Could you check a few things on this model? Use its own coordinates, in mm. Face numbers are marked on the shaded views. A direction names the side the tool comes from. Give positions to 0.01 mm unless a question says otherwise; leave off trailing zeros. Order: outer loops, then holes, each group sorted by start corner. A loop starts at its lowest first (then second) coordinate and runs counter-clockwise, first axis right, second up. Notation, with made-up numbers: (9, 45) -> (54, 45) arc R20 ccw to (54, 58) -> close; hole circle Ø3 at (-8.75, 49.5). An arc over 180 degrees is marked (long way). Answer as CSV lines item,"result". Start each with the question number.
(1) Will this pin go through, and if not, where does the flat tip stop? pin 1 Ø5 at (x, y) = (24, -1.5) entering from -Z.
(2) On a 3-axis mill with a long thin cutter (end or side, diameter ignored), from which of +Z, -Z, +X, -X, +Y, -Y can I reach the whole of each face in a straight line? I mean the marked faces 4 and 5. Say none if no direction works.
(3) I want a section at A-A (x = -8.5). Please give me the cut outline in (y, z).
(4) I want a section at C-C (z = 8.5). Please give me the cut outline in (x, y), plus the area to 4 significant figures.
(5) I want a section at B-B (y = -2). Please give me the cut outline in (x, z).
(6) We'd pull the mould along X, two halves only. Please class the marked faces 1, 2 and 3: released by +X, released by -X, zero draft, split by the parting line, or undercut.
(7) I need wall thicknesses on L1, parallel to X at y = 1, z = 2.75; L2, parallel to X at y = 6, z = 6; L3, parallel to Y at x = -19.5, z = 2. Which ranges of each line are inside material? Lowest first, please.
```python
from build123d import *

# Parameters (mm, degrees)
F0_W     = 67
F0_H     = 20
F0_W_2   = 5
F0_H_2   = 9
F0_H_3   = 10.5
F1_DEPTH = 10


with BuildPart() as f1:
    # F0 (on Top) → F1 (new body)
    with BuildSketch(Plane.XY):
        with Locations((2.5, 1.031276)):
            Rectangle(F0_W, F0_H)
        with Locations((26.5, 0.531276)):
            Rectangle(F0_W_2, F0_H_2, mode=Mode.SUBTRACT)
        with Locations((-21.5, 1.281276)):
            Rectangle(F0_W_2, F0_H_3, mode=Mode.SUBTRACT)
        with Locations((-9.5, 1.281276)):
            Rectangle(F0_W_2, F0_H_3, mode=Mode.SUBTRACT)
        with Locations((2.5, 1.281276)):
            Rectangle(F0_W_2, F0_H_3, mode=Mode.SUBTRACT)
        with Locations((14.5, 1.281276)):
            Rectangle(F0_W_2, F0_H_3, mode=Mode.SUBTRACT)
    extrude(amount=F1_DEPTH)


solid = f1.part
```
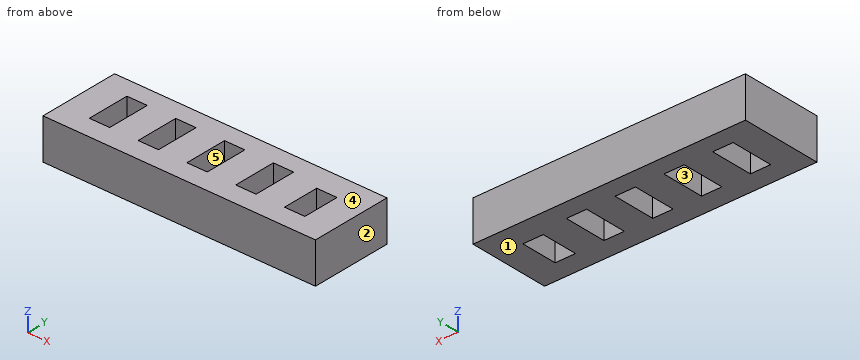
Final values:
1,pin 1,"z = 0"
2,face 4,"+Z, +X, -X, +Y, -Y"
2,face 5,"+Z, -Z"
3,outline,"(-8.97, 0) -> (-3.97, 0) -> (-3.97, 10) -> (-8.97, 10) -> close; (6.53, 0) -> (11.03, 0) -> (11.03, 10) -> (6.53, 10) -> close"
4,outline,"(-31, -8.97) -> (36, -8.97) -> (36, 11.03) -> (-31, 11.03) -> close; hole (-24, -3.97) -> (-19, -3.97) -> (-19, 6.53) -> (-24, 6.53) -> close; hole (-12, -3.97) -> (-7, -3.97) -> (-7, 6.53) -> (-12, 6.53) -> close; hole (0, -3.97) -> (5, -3.97) -> (5, 6.53) -> (0, 6.53) -> close; hole (12, -3.97) -> (17, -3.97) -> (17, 6.53) -> (12, 6.53) -> close; hole (24, -3.97) -> (29, -3.97) -> (29, 5.03) -> (24, 5.03) -> close"
4,area,"1,085 mm²"
5,outline,"(-31, 0) -> (-24, 0) -> (-24, 10) -> (-31, 10) -> close; (-19, 0) -> (-12, 0) -> (-12, 10) -> (-19, 10) -> close; (-7, 0) -> (0, 0) -> (0, 10) -> (-7, 10) -> close; (5, 0) -> (12, 0) -> (12, 10) -> (5, 10) -> close; (17, 0) -> (24, 0) -> (24, 10) -> (17, 10) -> close; (29, 0) -> (36, 0) -> (36, 10) -> (29, 10) -> close"
6,face 1,"zero draft"
6,face 2,"released by +X"
6,face 3,"undercut"
7,L1,"-31 to -24, -19 to -12, -7 to 0, 5 to 12, 17 to 24, 29 to 36"
7,L2,"-31 to -24, -19 to -12, -7 to 0, 5 to 12, 17 to 36"
7,L3,"-8.97 to -3.97, 6.53 to 11.03"
